Part model, mm, in its own coordinate system. Round coordinates to 2 decimals unless told otherwise and drop trailing zeros. Write each loop counter-clockwise with the first axis right and the second up, starting at its lowest first coordinate (ties: lowest second). Pieces come first, ordered by that corner, then holes.
```python
from build123d import *

# Parameters (mm, degrees)
SKETCH1_W           = 609.6
SKETCH1_H           = 393.7
BOSS_EXTRUDE1_DEPTH = 6.35


with BuildPart() as part:
    # Sketch1 → Boss-Extrude1 (new body)
    with BuildSketch(Plane(origin=(0, 0, 0), x_dir=(1, 0, 0), z_dir=(0, 1, 0))):
        with Locations((304.8, 196.85)):
            Rectangle(SKETCH1_W, SKETCH1_H)
        with BuildLine():
            Line((587.8, 32.05), (587.8, 17.05))
            ThreePointArc((587.8, 17.05), (584.8, 14.05), (581.8, 17.05))
            Line((581.8, 17.05), (581.8, 32.05))
            ThreePointArc((581.8, 32.05), (584.8, 35.05), (587.8, 32.05))
        make_face(mode=Mode.SUBTRACT)
        with BuildLine():
            Line((527.8, 32.05), (527.8, 17.05))
            ThreePointArc((527.8, 17.05), (524.8, 14.05), (521.8, 17.05))
            Line((521.8, 17.05), (521.8, 32.05))
            ThreePointArc((521.8, 32.05), (524.8, 35.05), (527.8, 32.05))
        make_face(mode=Mode.SUBTRACT)
        with BuildLine():
            Line((467.8, 32.05), (467.8, 17.05))
            ThreePointArc((467.8, 17.05), (464.8, 14.05), (461.8, 17.05))
            Line((461.8, 17.05), (461.8, 32.05))
            ThreePointArc((461.8, 32.05), (464.8, 35.05), (467.8, 32.05))
        make_face(mode=Mode.SUBTRACT)
        with BuildLine():
            Line((407.8, 32.05), (407.8, 17.05))
            ThreePointArc((407.8, 17.05), (404.8, 14.05), (401.8, 17.05))
            Line((401.8, 17.05), (401.8, 32.05))
            ThreePointArc((401.8, 32.05), (404.8, 35.05), (407.8, 32.05))
        make_face(mode=Mode.SUBTRACT)
        with BuildLine():
            Line((347.8, 32.05), (347.8, 17.05))
            ThreePointArc((347.8, 17.05), (344.8, 14.05), (341.8, 17.05))
            Line((341.8, 17.05), (341.8, 32.05))
            ThreePointArc((341.8, 32.05), (344.8, 35.05), (347.8, 32.05))
        make_face(mode=Mode.SUBTRACT)
        with BuildLine():
            Line((287.8, 32.05), (287.8, 17.05))
            ThreePointArc((287.8, 17.05), (284.8, 14.05), (281.8, 17.05))
            Line((281.8, 17.05), (281.8, 32.05))
            ThreePointArc((281.8, 32.05), (284.8, 35.05), (287.8, 32.05))
        make_face(mode=Mode.SUBTRACT)
        with BuildLine():
            Line((227.8, 32.05), (227.8, 17.05))
            ThreePointArc((227.8, 17.05), (224.8, 14.05), (221.8, 17.05))
            Line((221.8, 17.05), (221.8, 32.05))
            ThreePointArc((221.8, 32.05), (224.8, 35.05), (227.8, 32.05))
        make_face(mode=Mode.SUBTRACT)
        with BuildLine():
            Line((167.8, 32.05), (167.8, 17.05))
            ThreePointArc((167.8, 17.05), (164.8, 14.05), (161.8, 17.05))
            Line((161.8, 17.05), (161.8, 32.05))
            ThreePointArc((161.8, 32.05), (164.8, 35.05), (167.8, 32.05))
        make_face(mode=Mode.SUBTRACT)
        with BuildLine():
            Line((107.8, 32.05), (107.8, 17.05))
            ThreePointArc((107.8, 17.05), (104.8, 14.05), (101.8, 17.05))
            Line((101.8, 17.05), (101.8, 32.05))
            ThreePointArc((101.8, 32.05), (104.8, 35.05), (107.8, 32.05))
        make_face(mode=Mode.SUBTRACT)
        with BuildLine():
            Line((47.8, 32.05), (47.8, 17.05))
            ThreePointArc((47.8, 17.05), (44.8, 14.05), (41.8, 17.05))
            Line((41.8, 17.05), (41.8, 32.05))
            ThreePointArc((41.8, 32.05), (44.8, 35.05), (47.8, 32.05))
        make_face(mode=Mode.SUBTRACT)
        with BuildLine():
            Line((527.8, 376.65), (527.8, 361.65))
            ThreePointArc((527.8, 361.65), (524.8, 358.65), (521.8, 361.65))
            Line((521.8, 361.65), (521.8, 376.65))
            ThreePointArc((521.8, 376.65), (524.8, 379.65), (527.8, 376.65))
        make_face(mode=Mode.SUBTRACT)
        with BuildLine():
            Line((467.8, 376.65), (467.8, 361.65))
            ThreePointArc((467.8, 361.65), (464.8, 358.65), (461.8, 361.65))
            Line((461.8, 361.65), (461.8, 376.65))
            ThreePointArc((461.8, 376.65), (464.8, 379.65), (467.8, 376.65))
        make_face(mode=Mode.SUBTRACT)
        with BuildLine():
            Line((407.8, 376.65), (407.8, 361.65))
            ThreePointArc((407.8, 361.65), (404.8, 358.65), (401.8, 361.65))
            Line((401.8, 361.65), (401.8, 376.65))
            ThreePointArc((401.8, 376.65), (404.8, 379.65), (407.8, 376.65))
        make_face(mode=Mode.SUBTRACT)
        with BuildLine():
            Line((347.8, 376.65), (347.8, 361.65))
            ThreePointArc((347.8, 361.65), (344.8, 358.65), (341.8, 361.65))
            Line((341.8, 361.65), (341.8, 376.65))
            ThreePointArc((341.8, 376.65), (344.8, 379.65), (347.8, 376.65))
        make_face(mode=Mode.SUBTRACT)
        with BuildLine():
            Line((287.8, 376.65), (287.8, 361.65))
            ThreePointArc((287.8, 361.65), (284.8, 358.65), (281.8, 361.65))
            Line((281.8, 361.65), (281.8, 376.65))
            ThreePointArc((281.8, 376.65), (284.8, 379.65), (287.8, 376.65))
        make_face(mode=Mode.SUBTRACT)
        with BuildLine():
            Line((227.8, 376.65), (227.8, 361.65))
            ThreePointArc((227.8, 361.65), (224.8, 358.65), (221.8, 361.65))
            Line((221.8, 361.65), (221.8, 376.65))
            ThreePointArc((221.8, 376.65), (224.8, 379.65), (227.8, 376.65))
        make_face(mode=Mode.SUBTRACT)
        with BuildLine():
            Line((167.8, 376.65), (167.8, 361.65))
            ThreePointArc((167.8, 361.65), (164.8, 358.65), (161.8, 361.65))
            Line((161.8, 361.65), (161.8, 376.65))
            ThreePointArc((161.8, 376.65), (164.8, 379.65), (167.8, 376.65))
        make_face(mode=Mode.SUBTRACT)
        with BuildLine():
            Line((107.8, 376.65), (107.8, 361.65))
            ThreePointArc((107.8, 361.65), (104.8, 358.65), (101.8, 361.65))
            Line((101.8, 361.65), (101.8, 376.65))
            ThreePointArc((101.8, 376.65), (104.8, 379.65), (107.8, 376.65))
        make_face(mode=Mode.SUBTRACT)
        with BuildLine():
            Line((47.8, 376.65), (47.8, 361.65))
            ThreePointArc((47.8, 361.65), (44.8, 358.65), (41.8, 361.65))
            Line((41.8, 361.65), (41.8, 376.65))
            ThreePointArc((41.8, 376.65), (44.8, 379.65), (47.8, 376.65))
        make_face(mode=Mode.SUBTRACT)
        with BuildLine():
            Line((587.8, 376.65), (587.8, 361.65))
            ThreePointArc((587.8, 361.65), (584.8, 358.65), (581.8, 361.65))
            Line((581.8, 361.65), (581.8, 376.65))
            ThreePointArc((581.8, 376.65), (584.8, 379.65), (587.8, 376.65))
        make_face(mode=Mode.SUBTRACT)
        with BuildLine():
            Line((506.85, 209.125), (556.85, 209.125))
            ThreePointArc((556.85, 209.125), (559.6, 206.375), (556.85, 203.625))
            Line((556.85, 203.625), (506.85, 203.625))
            ThreePointArc((506.85, 203.625), (504.1, 206.375), (506.85, 209.125))
        make_face(mode=Mode.SUBTRACT)
        with BuildLine():
            Line((506.85, 190.075), (556.85, 190.075))
            ThreePointArc((556.85, 190.075), (559.6, 187.325), (556.85, 184.575))
            Line((556.85, 184.575), (506.85, 184.575))
            ThreePointArc((506.85, 184.575), (504.1, 187.325), (506.85, 190.075))
        make_face(mode=Mode.SUBTRACT)
    extrude(amount=BOSS_EXTRUDE1_DEPTH)


solid = part.part
```
Q1. Wall check: L1, parallel to Z at x = 549, y = 4.5 (3 decimals); L2, parallel to Z at x = 164.5, y = 4. Give the ranges that are in metal, low to high.
Values follow:
L1: z = -393.7 to -209.125, -203.625 to -190.075, -184.575 to 0
L2: z = -393.7 to -379.63, -358.67 to -35.03, -14.07 to 0
Q2. Drop a flat-ended pin along its axis: pin 1 (2 mm diameter, centred on x = 287.5, z = -323, fed in from -Y). Give the stop position or say it passes through.
Values follow:
pin 1: stops at y = 0
Q3. Cut at A-A on x = 544.5. Write the cut outline in (y, z) (3 decimals), plus the area to 3 significant figures.
Values follow:
outline: (0, -393.7) - (6.35, -393.7) - (6.35, -209.125) - (0, -209.125) - close; (0, -203.625) - (6.35, -203.625) - (6.35, -190.075) - (0, -190.075) - close; (0, -184.575) - (6.35, -184.575) - (6.35, 0) - (0, 0) - close
area: 2,430 mm2
